```python
from build123d import *

# Parameters (mm, degrees)
F0_R      = 2
F1_DEPTH  = 9
F2_DEPTH  = 13
F4_DEPTH  = 5
F6_DEPTH  = 8.001
F7_R      = 4.99999
F8_R      = 5
F9_R      = 5
F10_R     = 4.05
F11_DEPTH = 14.001


# Not quite as in the source:
# - a fillet or chamfer is up to 0.001 mm smaller than in the source, because OpenCascade refuses the exact size


with BuildPart() as f1:
    # F0 (on Top) → F1 (new body)
    with BuildSketch(Plane.XY):
        Polygon((8.7753673922, -59.6295086741), (-35.2246326078, -59.6295086741), (-35.2246326078, -64.6295086741), (-6.2246326078, -64.6295086741), (-6.2246326078, -69.6295086741), (3.7753673922, -69.6295086741), (3.7753673922, -109.6295086741), (-6.2246326078, -109.6295086741), (-6.2246326078, -119.6295086741), (8.7753673922, -119.6295086741), align=None)
        with Locations((-1.2246326078, -114.6295086741)):
            Circle(F0_R, mode=Mode.SUBTRACT)
        with Locations((-1.2246326078, -64.6295086741)):
            Circle(F0_R, mode=Mode.SUBTRACT)
    extrude(amount=F1_DEPTH)

    # F0 (on Top) → F2 (join)
    with BuildSketch(Plane.XY):
        Polygon((-21.2246326078, 61.3704913259), (-21.2246326078, 91.3704913259), (-35.2246326078, 91.3704913259), (-35.2246326078, -59.6295086741), (8.7753673922, -59.6295086741), (8.7753673922, -49.6295086741), align=None)
    extrude(amount=F2_DEPTH)

    # F3 (on face) → F4 (cut)
    with BuildSketch(Plane.XY.offset(13)):
        Polygon((2.6947563819, -38.6295086741), (-24.3322706451, 61.3704913259), (-32.2246326078, 61.3704913259), (-32.2246326078, -38.6295086741), align=None)
    extrude(amount=-F4_DEPTH, mode=Mode.SUBTRACT)

    # F5 (on face) → F6 (cut, through all)
    with BuildSketch(Plane.XY.offset(8)):
        Polygon((-26.6290978716, 58.3704913259), (-29.2246326078, 58.3704913259), (-29.2246326078, 36.3704913259), (-20.6831519256, 36.3704913259), align=None)
        Polygon((-19.8723411148, 33.3704913259), (-29.2246326078, 33.3704913259), (-29.2246326078, 11.3704913259), (-16.7414328131, 21.7861306095), align=None)
        Polygon((-15.879765316, 18.5979608701), (-29.2246326078, 7.463369877), (-29.2246326078, 2.463369877), (-7.3999758243, -12.777260249), align=None)
        Polygon((-6.1809639439, -17.2876042066), (-29.2246326078, -1.1957117047), (-29.2246326078, -35.6295086741), (-1.2236924662, -35.6295086741), align=None)
    extrude(amount=-F6_DEPTH, mode=Mode.SUBTRACT)

    # F7 (radius 5 in the source; OpenCascade refuses exactly that, so slightly less here)
    f7_edges = [f1.edges().sort_by_distance(p)[0] for p in [
        (-6.224633, -69.629509, 4.5),
    ]]
    fillet(f7_edges, radius=F7_R)

    # F8
    f8_edges = [f1.edges().sort_by_distance(p)[0] for p in [
        (-6.224633, -109.629509, 4.5),
    ]]
    fillet(f8_edges, radius=F8_R)

    # F9
    f9_edges = [f1.edges().sort_by_distance(p)[0] for p in [
        (-35.224633, -64.629509, 4.5),
    ]]
    fillet(f9_edges, radius=F9_R)

    # F10 (on face) → F11 (cut, through all)
    with BuildSketch(Plane.YZ.offset(-21.2246326078)):
        with Locations((85.3704913259, 6.5)):
            Circle(F10_R)
    extrude(amount=-F11_DEPTH, mode=Mode.SUBTRACT)


solid = f1.part
```
Source: CAD feature listing. Evaluate the final solid. Frame: model axes, mm. A direction names the side the tool comes from. Give positions to 0.01 mm unless a question says otherwise; leave off trailing zeros. Write each loop counter-clockwise with the first axis right and the second up, starting at its lowest first coordinate (ties: lowest second). Pieces come first, ordered by that corner, then holes.
1. Section query D-D (y = -46). Return the cut outline in (x, z), then the cut area to 3 significant figures.
2. Access query for faces 4 (the face through (3.775, -89, 4)), 5 (the face through (-35.225, 17, 6)), 6 (the face through (-15, -35.63, 4)), 7 (the face through (5, -81, 9)), 8 (the face through (-32.225, 12, 11)). Directions: +Z, -Z, +X, -X, +Y, -Y. A direction counts if a zero-diameter tool reaches every point of the face in a straight line with its end or side. Return the directions, or none.
3. First-contact query: pin 1 (6.5 mm diameter, centred on x = -1.22, y = -114.63, fed in from +Z); pin 2 (8 mm diameter, centred on x = -29, y = 17.5, fed in from +Z); pin 3 (2.5 mm diameter, centred on y = 4.5, z = 4.5, fed in from +X); pin 4 (6.5 mm diameter, centred on y = 50.5, z = 2.5, fed in from +X). Flat tips, straight axial feed; report the tip coordinate or a pass-through.
4. Section query B-B (y = 48). Return the cut outline in (x, z), then the cut area to 3 significant figures.
5. Section query A-A (x = -11). Return the cut outline in (y, z), then the cut area to 3 significant figures.
6. Section query C-C (y = -97). Return the cut outline in (x, z).
7. Pull-direction query (Y, two-part tool) for faces 1 (the face through (-6.015, 5.093, 6.409)), 2 (the face through (-28, 61.37, 11)), 3 (the face through (-6.225, -117, 4)); classes: +Y half, -Y half, draft (parallel to the pull), parting line (faces both ways), or undercut.
8. Material intervals for line 1 along Y through (x, z) = (-28.5, 4); line 2 along X through (y, z) = (71, 9.75); line 3 along Z through (x, y) = (7.5, -84), sorted ascending.
Output values:
1. outline: (-35.22, 0) - (7.79, 0) - (7.79, 13) - (-35.22, 13) - close
1. area: 559 mm2
2. face 4: +Z, -Z, -X
2. face 5: +Z, -Z, -X, +Y, -Y
2. face 6: +Z, -Z
2. face 7: +Z, +X, -X, -Y
2. face 8: +Z
3. pin 1: stops at z = 9
3. pin 2: stops at z = 13
3. pin 3: stops at x = -5.52
3. pin 4: stops at x = -17.41
4. outline: (-35.22, 0) - (-29.22, 0) - (-29.22, 8) - (-32.22, 8) - (-32.22, 13) - (-35.22, 13) - close; (-23.83, 0) - (-17.61, 0) - (-17.61, 13) - (-20.72, 13) - (-20.72, 8) - (-23.83, 8) - close
4. area: 128 mm2
5. outline: (-64.63, 0) - (-35.63, 0) - (-35.63, 8) - (-38.63, 8) - (-38.63, 13) - (-59.63, 13) - (-59.63, 9) - (-64.63, 9) - close; (-13.92, 0) - (-10.26, 0) - (-10.26, 8) - (-13.92, 8) - close; (0.54, 0) - (23.54, 0) - (23.54, 13) - (12.04, 13) - (12.04, 8) - (0.54, 8) - close
5. area: 613 mm2
6. outline: (3.78, 0) - (8.78, 0) - (8.78, 9) - (3.78, 9) - close
7. face 1: +Y half
7. face 2: undercut
7. face 3: draft
8. line 1: y = -64.63 to -35.63, -1.7 to 1.96, 8.07 to 11.98, 33.37 to 36.37, 58.37 to 82.18, 88.56 to 91.37
8. line 2: x = -35.22 to -21.22
8. line 3: z = 0 to 9
